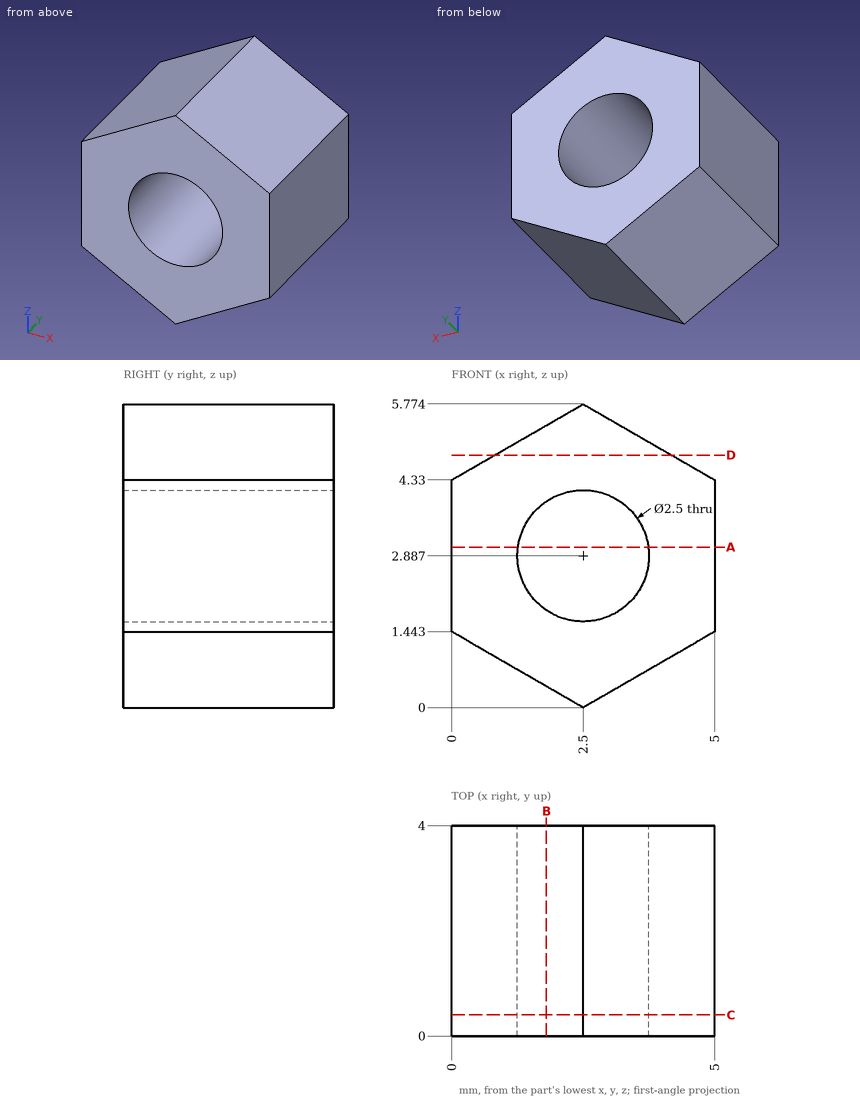
Study the drawing (mm; zero at the part's minimum x, y, z) and answer. Give positions to 0.01 mm unless a question says otherwise; leave off trailing zeros. Loops run counter-clockwise (first coordinate to the right, second up) from the corner with the lowest first, then second, coordinate; pieces in that order, holes last. Notation, with made-up numbers: (15, -32) - (72, -32) arc R32 cw to (72, -2) - close; hole circle Ø11 at (25, 30). An arc over 180 degrees is marked (long way). Return JSON: item names as keys, results as strings. Group by question number.
1. Find section B-B (x = 1.8). Write down the section's boundary in (y, z) (1 decimal).
2. Find section C-C (y = 0.4). Write down the section's boundary in (x, z).
3. Find section A-A (z = 3.05). Write down the section's boundary in (x, y).
4. Straight lines are drawn through the part: line 1 (X direction, y = 0.55, z = 2.1); line 2 (X direction, y = 1.5, z = 3.85) (1 decimal); line 3 (Z direction, x = 2.3, y = 3.8) (1 decimal). For each, find the intervals that lie inside material, in ascending order. Write a range as [from, to].
5. Find section D-D (z = 4.8). Write down the section's boundary in (x, y).
Verdict:
{
 "1": {"outline": "(0, 0.4) - (4, 0.4) - (4, 1.9) - (0, 1.9) - close; (0, 3.9) - (4, 3.9) - (4, 5.4) - (0, 5.4) - close"},
 "2": {"outline": "(0, 1.44) - (2.5, 0) - (5, 1.44) - (5, 4.33) - (2.5, 5.77) - (0, 4.33) - close; hole circle Ø2.5 at (2.5, 2.89)"},
 "3": {"outline": "(0, 0) - (1.26, 0) - (1.26, 4) - (0, 4) - close; (3.74, 0) - (5, 0) - (5, 4) - (3.74, 4) - close"},
 "4": {"line 1": "x = [0, 1.53], [3.47, 5]", "line 2": "x = [0, 1.7], [3.3, 5]", "line 3": "z = [0.1, 1.7], [4.1, 5.7]"},
 "5": {"outline": "(0.81, 0) - (4.19, 0) - (4.19, 4) - (0.81, 4) - close"}
}
